Source: CAD feature listing. Evaluate the final solid. Frame: model axes, mm. Face numbers are marked on the shaded views. A direction names the side the tool comes from. Give positions to 0.01 mm unless a question says otherwise; leave off trailing zeros. Loops run counter-clockwise (first coordinate to the right, second up) from the corner with the lowest first, then second, coordinate; pieces in that order, holes last. Notation, with made-up numbers: (3.5, 9) - (40.5, 9) arc R26 cw to (40.5, 46) - close; hole circle Ø2 at (27.5, 58). An arc over 180 degrees is marked (long way). Write each question's results on one line, items separated by ' | '. Start each with the question number.
(1) Reachability of the marked faces 3, 4 and 5 from +Z, -Z, +X, -X, +Y, -Y: full face, straight path, thin tool, end or side. Return the list, or none.
(2) Material intervals for line 1 along X through (y, z) = (5.5, 3.25); line 2 along X through (y, z) = (7, 10.5); line 3 along Y through (x, z) = (-76, 6.5) (3 decimals), sorted ascending. Write a range as [from, to].
(3) Cut plane C-C on x = -28.5. Return the cut outline in (y, z) (3 decimals).
(4) Pull-direction query (X, two-part tool) for the marked faces 1 and 2; classes: pulls with the +X half, pulls with the -X half, needs draft (parallel to the pull), parting line crosses it, or undercut.
(5) Cut plane B-B on y = 10. Return the cut outline in (x, z).
(6) Contact query for flat-ended pins moving along their axis: pin 1 (6.5 mm diameter, centred on x = -16.5, z = 8.5, fed in from +Y) (3 decimals); pin 2 (7 mm diameter, centred on y = 11, z = 7, fed in from +X); pin 3 (5 mm diameter, centred on y = 9.5, z = 7.5, fed in from -X). Output: stop coordinate, or through.
(7) Cut plane A-A on z = 8.5. Return the cut outline in (x, y) (3 decimals), then the cut area to 3 significant figures.
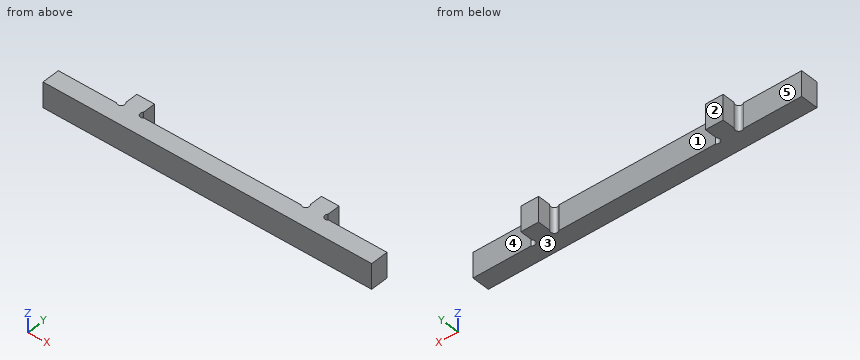
from build123d import *

# Parameters (mm, degrees)
BOSS_EXTRUDE1_DEPTH = 12.7


with BuildPart() as part:
    # Sketch1 → Boss-Extrude1 (new body)
    with BuildSketch(Plane.XY):
        with BuildLine():
            Line((-53.34, 4.445), (-82.55, 4.445))
            Line((-82.55, 4.445), (-82.55, -4.445))
            Line((-82.55, -4.445), (82.55, -4.445))
            Line((82.55, -4.445), (82.55, 4.445))
            Line((82.55, 4.445), (53.34, 4.445))
            ThreePointArc((53.34, 4.445), (50.8, 4.445), (50.8, 6.985))
            Line((50.8, 6.985), (50.8, 13.335))
            Line((50.8, 13.335), (41.91, 13.335))
            Line((41.91, 13.335), (41.91, 6.985))
            ThreePointArc((41.91, 6.985), (41.91, 4.445), (39.37, 4.445))
            Line((39.37, 4.445), (-39.37, 4.445))
            ThreePointArc((-39.37, 4.445), (-41.91, 4.445), (-41.91, 6.985))
            Line((-41.91, 6.985), (-41.91, 13.335))
            Line((-41.91, 13.335), (-50.8, 13.335))
            Line((-50.8, 13.335), (-50.8, 6.985))
            ThreePointArc((-50.8, 6.985), (-50.8, 4.445), (-53.34, 4.445))
        make_face()
    extrude(amount=BOSS_EXTRUDE1_DEPTH)


solid = part.part
Ans:
1) face 3: -Z, +X, -X, +Y, -Y | face 4: +Z, -Z, +X, +Y | face 5: +Z, -Z, -X, +Y
2) line 1: [-50.29, -42.42], [42.42, 50.29] | line 2: [-50.8, -41.91], [41.91, 50.8] | line 3: [-4.445, 4.445]
3) outline: (-4.445, 0) - (4.445, 0) - (4.445, 12.7) - (-4.445, 12.7) - close
4) face 1: undercut | face 2: needs draft
5) outline: (-50.8, 0) - (-41.91, 0) - (-41.91, 12.7) - (-50.8, 12.7) - close; (41.91, 0) - (50.8, 0) - (50.8, 12.7) - (41.91, 12.7) - close
6) pin 1: y = 4.445 | pin 2: x = 50.8 | pin 3: x = -50.8
7) outline: (-82.55, -4.445) - (82.55, -4.445) - (82.55, 4.445) - (53.34, 4.445) arc R1.796 cw to (50.8, 6.985) - (50.8, 13.335) - (41.91, 13.335) - (41.91, 6.985) arc R1.796 cw to (39.37, 4.445) - (-39.37, 4.445) arc R1.796 cw to (-41.91, 6.985) - (-41.91, 13.335) - (-50.8, 13.335) - (-50.8, 6.985) arc R1.796 cw to (-53.34, 4.445) - (-82.55, 4.445) - close | area: 1,620 mm^2
